Check sheet for the drawn part. Datum: minimum x, y, z corner. Units: mm. A direction names the side the tool comes from. Give positions to 0.01 mm unless a question says otherwise; leave off trailing zeros. Order: outer loops, then holes, each group sorted by start corner. A loop starts at its lowest first (then second) coordinate and runs counter-clockwise, first axis right, second up. Notation, with made-up numbers: (55.25, 23.25) -> (67.25, 23.25) arc R19 ccw to (67.25, 34.25) -> close; hole circle Ø1 at (-18, 34). An arc over 180 degrees is marked (long way). One line per question, with ' | ' between items. Start each with the question number.
Q1. Material ranges on probe 1 along Y at (x, z) = (6.5, 7.25); probe 2 along X at (y, z) = (13.25, 10); probe 3 along X at (y, z) = (12.25, 10.5), recorded low to high. Write a range as [from, to].
Q2. Section check C-C on y = 12.5. Record the cut outline in (x, z), plus the area to 3 significant figures.
Q3. Mould release check, pull along X, two halves, no side actions. Record for the marked faces 3, 4, 5 and 6: released by +X, released by -X, zero draft, split by the parting line, or undercut.
Q4. Section check B-B on z = 8.75. Record the cut outline in (x, y).
Q5. Section check A-A on x = 8.75. Record the cut outline in (y, z).
Q6. Go/stop test with flat-tipped pins: pin 1 (0.9 mm diameter, centred on x = 9, y = 13, fed in from -Z); pin 2 (5 mm diameter, centred on y = 6.5, z = 13.5, fed in from -X); pin 3 (5 mm diameter, centred on x = 6, y = 12.5, fed in from +Z). Record where each tip stops, or that it passes through.
Q7. Section check D-D on y = 8. Record the cut outline in (x, z), plus the area to 3 significant figures.
Q8. Access from +Z, -Z, +X, -X, +Y, -Y to the whole of each face (thin tool, end or side, straight path). Record for the marked faces 1 and 2.
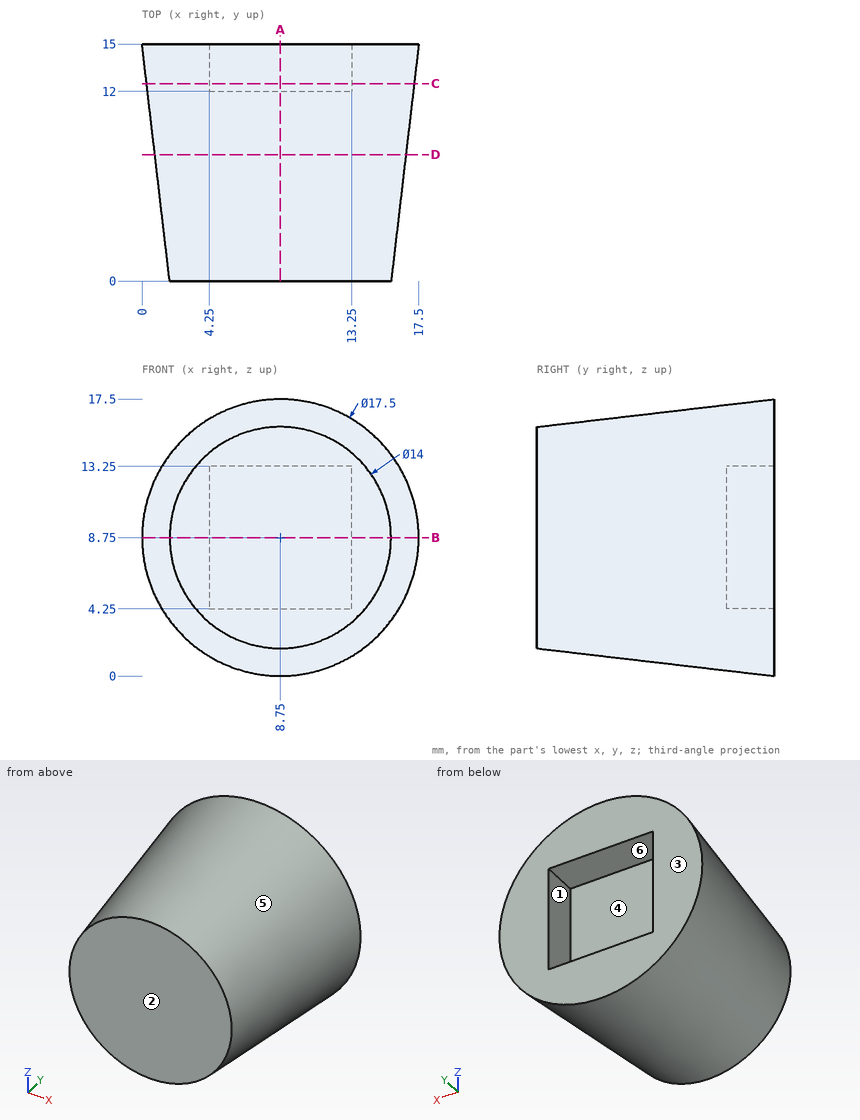
Filled in:
1) probe 1: [0, 12] | probe 2: [0.3, 4.25], [13.25, 17.2] | probe 3: [0.5, 4.25], [13.25, 17]
2) outline: circle Ø16.92 at (8.75, 8.75); hole (4.25, 4.25) -> (13.25, 4.25) -> (13.25, 13.25) -> (4.25, 13.25) -> close | area: 144 mm²
3) face 3: zero draft | face 4: undercut | face 5: split by the parting line | face 6: undercut
4) outline: (0, 15) -> (1.75, 0) -> (15.75, 0) -> (17.5, 15) -> (13.25, 15) -> (13.25, 12) -> (4.25, 12) -> (4.25, 15) -> close
5) outline: (0, 1.75) -> (15, 0) -> (15, 4.25) -> (12, 4.25) -> (12, 13.25) -> (15, 13.25) -> (15, 17.5) -> (0, 15.75) -> close
6) pin 1: z = 0.18 | pin 2: x = 1.27 | pin 3: z = 17.36
7) outline: circle Ø15.87 at (8.75, 8.75) | area: 198 mm²
8) face 1: +Y | face 2: +Z, -Z, +X, -X, -Y
